```python
from build123d import *

# Parameters (mm, degrees)
ESQUISSE1_W             = 30
ESQUISSE1_H             = 80
BOSS_EXTRU_1_DEPTH      = 3
ESQUISSE2_R             = 2.125
ENL_V_MAT_EXTRU_1_DEPTH = 3
ESQUISSE3_W             = 30
ESQUISSE3_H             = 30
BOSS_EXTRU_2_DEPTH      = 5
BOSS_EXTRU_3_DEPTH      = 30
CONG_1_R                = 1
CONG_2_R                = 2.5


with BuildPart() as part:
    # Esquisse1 → Boss.-Extru.1 (new body)
    with BuildSketch(Plane.XY):
        with Locations((15, 40)):
            Rectangle(ESQUISSE1_W, ESQUISSE1_H)
    extrude(amount=BOSS_EXTRU_1_DEPTH)

    # Esquisse2 → Enlèv. mat.-Extru.1 (cut)
    with BuildSketch(Plane.XY.offset(3)):
        with Locations((15, 67.5)):
            Circle(ESQUISSE2_R)
        with Locations((15, 12.5)):
            Circle(ESQUISSE2_R)
    extrude(amount=-ENL_V_MAT_EXTRU_1_DEPTH, mode=Mode.SUBTRACT)

    # Esquisse3 → Boss.-Extru.2 (add)
    with BuildSketch(Plane.XY.offset(3)):
        with Locations((15, 40)):
            Rectangle(ESQUISSE3_W, ESQUISSE3_H)
    extrude(amount=BOSS_EXTRU_2_DEPTH)

    # Esquisse4 → Boss.-Extru.3 (add)
    with BuildSketch(Plane(origin=(0, 25, 0), x_dir=(-1, 0, 0), z_dir=(0, -1, 0))):
        Polygon((-12.5, -8), (-12.5, -10), (-9, -10), (-9, -11.81), (-12.75, -13.201941091), (-17.25, -13.201941091), (-21, -11.81), (-21, -10), (-17.5, -10), (-17.5, -8), align=None)
    extrude(amount=-BOSS_EXTRU_3_DEPTH)

    # Congé1
    cong_1_edges = [part.edges().sort_by_distance(p)[0] for p in [
        (9, 40, 10),
        (9, 40, 11.81),
        (12.75, 40, 13.201941091),
        (17.25, 40, 13.201941091),
        (21, 40, 11.81),
        (21, 40, 10),
    ]]
    fillet(cong_1_edges, radius=CONG_1_R)

    # Congé2
    cong_2_edges = [part.edges().sort_by_distance(p)[0] for p in [
        (15, 55, 3),
        (15, 25, 3),
    ]]
    fillet(cong_2_edges, radius=CONG_2_R)
    cong_2_2_edges = [part.edges().sort_by_distance(p)[0] for p in [
        (0, 0, 1.5),
        (30, 40, 8),
        (0, 40, 8),
        (30, 80, 1.5),
        (0, 80, 1.5),
        (15, 80, 3),
        (30, 68.75, 3),
        (0, 68.75, 3),
        (30, 0, 1.5),
        (15, 0, 3),
        (0, 11.25, 3),
        (30, 11.25, 3),
        (23.75, 25, 8),
        (6.25, 25, 8),
        (23.75, 55, 8),
        (6.25, 55, 8),
        (30, 24.267766953, 3.732233047),
        (0, 24.267766953, 3.732233047),
        (0, 55.732233047, 3.732233047),
        (30, 55.732233047, 3.732233047),
    ]]
    fillet(cong_2_2_edges, radius=CONG_2_R - 0.0001)  # a hair under: the kernel refuses the full size


solid = part.part
```
CAD build for the part. Positions are in the model's coordinates, mm. A direction names the side the tool comes from. Give positions to 0.01 mm unless a question says otherwise; leave off trailing zeros. Loops run counter-clockwise (first coordinate to the right, second up) from the corner with the lowest first, then second, coordinate; pieces in that order, holes last. Notation, with made-up numbers: (60, 7) - (76, 7) arc R14 cw to (76, 21) - close; hole circle Ø3 at (86, 47.25). An arc over 180 degrees is marked (long way). Put each result on its own line as item: value.
Q1. Flat gauge pins, fed straight in: pin 1 (2.5 mm diameter, centred on x = 11, z = 9, fed in from -Y); pin 2 (16 mm diameter, centred on x = 12, y = 11.5, fed in from +Z); pin 3 (2 mm diameter, centred on y = 41.5, z = 7, fed in from -X). Where does each tip first touch, or does it go through?
Filled in:
pin 1: stops at y = 25
pin 2: stops at z = 3
pin 3: stops at x = 0.05
Q2. Slice it at A-A (x = 15). Give the cut face in (y, z) (3 decimals), plus the area to 3 significant figures.
Filled in:
outline: (0, 0) - (10.375, 0) - (10.375, 3) - (2.5, 3) arc R2.5 ccw to (0, 0.5) - close; (14.625, 0) - (65.375, 0) - (65.375, 3) - (57.5, 3) arc R2.5 cw to (55, 5.5) - (55, 13.202) - (25, 13.202) - (25, 5.5) arc R2.5 cw to (22.5, 3) - (14.625, 3) - close; (69.625, 0) - (80, 0) - (80, 0.5) arc R2.5 ccw to (77.5, 3) - (69.625, 3) - close
area: 521 mm²
Q3. Mould opens along X. For faces 6 (the face through (17.5, 40, 9)), 7 (the face through (7.57, 54.248, 7.287)), 8 (the face through (12.877, 12.593, 1.521)) say: pulls with the +X half, pulls with the -X half, needs draft (parallel to the pull), parting line crosses it, or undercut.
Filled in:
face 6: pulls with the +X half
face 7: needs draft
face 8: undercut
Q4. Probe line 1 along Y through (x, z) = (15, 0.75) (3 decimals); line 2 along Y through (x, z) = (15, 2) (3 decimals); line 3 along X through (y, z) = (34, 8.25). List the from-to ranges inside material, lowest first.
Filled in:
line 1: y = 0.013 to 10.375, 14.625 to 65.375, 69.625 to 79.987
line 2: y = 0.5 to 10.375, 14.625 to 65.375, 69.625 to 79.5
line 3: x = 12.5 to 17.5
Q5. Tool access for faces 1 (the face through (19, 40, 10)), 2 (the face through (29.287, 12.64, 2.248)), 3 (the face through (15, 55, 10)), 4 (the face through (7, 40, 8)), 5 (the face through (22.57, 25.713, 7.248)): list every direction of +Z, -Z, +X, -X, +Y, -Y with a clear straight run to the whole face (end or side of a thin tool).
Filled in:
face 1: +X, +Y, -Y
face 2: +Z, +X, -Y
face 3: +Z, +X, -X, +Y
face 4: -X, +Y, -Y
face 5: +X, -Y
Q6. Slice it at C-C (y = 44.5). Give the cut face in (x, z), plus the area to 3 significant figures.
Filled in:
outline: (0, 0) - (30, 0) - (30, 5.5) arc R2.5 ccw to (27.5, 8) - (17.5, 8) - (17.5, 10) - (20, 10) arc R1 ccw to (21, 11) - (21, 11.11) arc R1 ccw to (20.35, 12.05) - (17.42, 13.14) arc R1 ccw to (17.07, 13.2) - (12.93, 13.2) arc R1 ccw to (12.58, 13.14) - (9.65, 12.05) arc R1 ccw to (9, 11.11) - (9, 11) arc R1 ccw to (10, 10) - (12.5, 10) - (12.5, 8) - (2.5, 8) arc R2.5 ccw to (0, 5.5) - close
area: 280 mm²
Q7. Slice it at B-B (y = 12.5). Give the cut face in (x, z) (3 decimals), plus the area to 3 significant figures.
Filled in:
outline: (0, 0) - (12.875, 0) - (12.875, 3) - (2.5, 3) arc R2.5 ccw to (0, 0.5) - close; (17.125, 0) - (30, 0) - (30, 0.5) arc R2.5 ccw to (27.5, 3) - (17.125, 3) - close
area: 74.6 mm²
